Read the model definition and answer for the solid it produces. Units are mm, in the model's axes. Face numbers are marked on the shaded views. A direction names the side the tool comes from. Coordinates: 2 decimals unless noted, no trailing zeros. Write each loop counter-clockwise with the first axis right and the second up, starting at its lowest first coordinate (ties: lowest second). Pieces come first, ordered by that corner, then holes. Notation, with made-up numbers: (70.5, 21) -> (107.5, 21) arc R18 cw to (107.5, 34) -> close; hole circle Ø1 at (87, 20). An arc over 180 degrees is marked (long way). One line per item, written item: value. Start each with the question number.
1. Consider line 1 along Y through (x, z) = (-31, 1025.5); line 2 along X through (y, z) = (78.5, 673); line 3 along Y through (x, z) = (-10, 243). Determine where each line is inside the solid, lowest interval first.
2. Find section C-C, the plane y = 4. Write down the section's boundary in (x, z).
3. Given P1, Ø1.5, axis at y = 58, z = 167, coming from the -X side; P2, Ø2, axis at y = -53.5, z = 1196, coming from the +X side; P3, Ø2, axis at x = -2.5, y = 19.5, coming from the -Z side, each flat-ended and moving along its own axis, determine where each tip first touches the part or whether it passes through.
4. Find section A-A, the plane x = 38.5. Write down the section's boundary in (y, z), and give its area (3 significant figures).
5. For the marked faces 1 and 2, determine the directions among +Z, -Z, +X, -X, +Y, -Y from which every point of the face is accessible in a straight line to the end or side of a thin tool.
6. Find section B-B, the plane z = 515. Write down the section's boundary in (x, y), and give its area (3 significant figures).
Autodesk Inventor part; units mm, degrees
ref_plane "Start plane" through (0, 0, 0) normal (0, 0, 1) x (1, 0, 0)
ref_plane "End plane" through (0, 0, 1500) normal (0, 0, 1) x (1, 0, 0)
ref_plane "Work Plane4" through (-55, 0, -55) normal (0.7071, 0, -0.7071) x (-0.7071, 0, -0.7071)
ref_plane "Start plane" through (0, 0, 0) normal (0, 0, 1) x (1, 0, 0)
ref_plane "End plane" through (0, 0, 1500) normal (0, 0, 1) x (1, 0, 0)
sketch "Sketch2" plane through (0, 0, 0) normal (0, 0, 1) x (1, 0, 0)
  line L0 (-55, 100.8) -> (-14.95, 100.8)
  line L1 (-55, 110) -> (-55, 100.8)
  line L2 (55, 110) -> (-55, 110)
  line L3 (55, 100.8) -> (55, 110)
  line L4 (14.95, 100.8) -> (55, 100.8)
  line L5 (2.95, -88.8) -> (2.95, 88.8)
  line L6 (55, -100.8) -> (14.95, -100.8)
  line L7 (55, -110) -> (55, -100.8)
  line L8 (-55, -100.8) -> (-55, -110)
  line L9 (-14.95, -100.8) -> (-55, -100.8)
  line L10 (-2.95, 88.8) -> (-2.95, -88.8)
  line L11 (0, -154) -> (0, 154) construction
  line L12 (-2.95, -100.8) -> (2.95, -100.8) construction
  arc A0 (-14.95, -100.8) -> (-2.95, -88.8) centre (-14.95, -88.8) ccw
  arc A1 (-2.95, 88.8) -> (-14.95, 100.8) centre (-14.95, 88.8) ccw
  arc A2 (14.95, 100.8) -> (2.95, 88.8) centre (14.95, 88.8) ccw
  arc A3 (2.95, -88.8) -> (14.95, -100.8) centre (14.95, -88.8) ccw
  line L13 (-77, 0) -> (77, 0) construction
  line L14 (-55, -110) -> (55, -110)
  point P0 (-2.95, 100.8)
  point P1 (2.95, 100.8)
  point P2 (0, 0)
  point P3 (0, -100.8)
  point P4 (0, 0)
  dimension "d1" = 220
  dimension "d3" = 9.2
  dimension "d5" = 5.9
  dimension "d7" = 110
  dimension "d13" = 12
  dimension "d14" = 110
  dimension "d15" = 55
extrude "Body" add sketch "Sketch2" along normal up to surface (1500 mm away) from surface at 0
sketch "Sketch3" plane through (0, 0, 0) normal (0, 0, 1) x (1, 0, 0)
  line L0 (0, 0) -> (10, 0)
ref_plane "Work Plane3" through (0, 0, 0) normal (0, -1, 0) x (1, 0, 0)
ref_plane "Work Plane4" through (-55, 0, -55) normal (0.7071, 0, -0.7071) x (-0.7071, 0, -0.7071)
split "Split1" plane through (-55, 0, -55) removes the side toward (0.7071, 0, -0.7071)
ref_plane "Work Plane5" through (55, 0, -55) normal (-0.7071, 0, -0.7071) x (-0.7071, 0, 0.7071)
split "Split2" plane through (55, 0, -55) removes the side toward (-0.7071, 0, -0.7071)
ref_plane "Work Plane6" through (55, 0, 1555) normal (-0.7071, 0, 0.7071) x (0.7071, 0, 0.7071)
split "Split3" plane through (55, 0, 1555) removes the side toward (-0.7071, 0, 0.7071)
ref_plane "Work Plane7" through (-55, 0, 1555) normal (0.7071, 0, 0.7071) x (0.7071, 0, -0.7071)
split "Split4" plane through (-55, 0, 1555) removes the side toward (0.7071, 0, 0.7071)
sketch "Sketch4" plane through (0, 0, 0) normal (0, -1, 0) x (1, 0, 0)
  line L0 (-2, 0) -> (12, 0)
  line L1 (-2, 1500) -> (12, 1500)
  dimension "d19" = 1500
equation "\"d1\" = ParH"
equation "\"d3\" = t2"
equation "\"d7\" = b"
equation "\"d13\" = R1"
equation "\"d14\" = 0.5 * d1"
equation "\"d15\" = 0.5 * d7"
equation "\"d8\" = G_L"
equation "\"b\" = 110"
equation "\"ParH\" = 220"
equation "\"R1\" = 12"
equation "\"G_L\" = d19"
equation "\"t1\" = 5.9"
equation "\"t2\" = 9.2"
equation "\"G_OFFSET_START\" = 0"
equation "\"G_OFFSET_END\" = 0"
properties part number "DIN 1025 - IPE 220-1500" material "Steel, Mild"
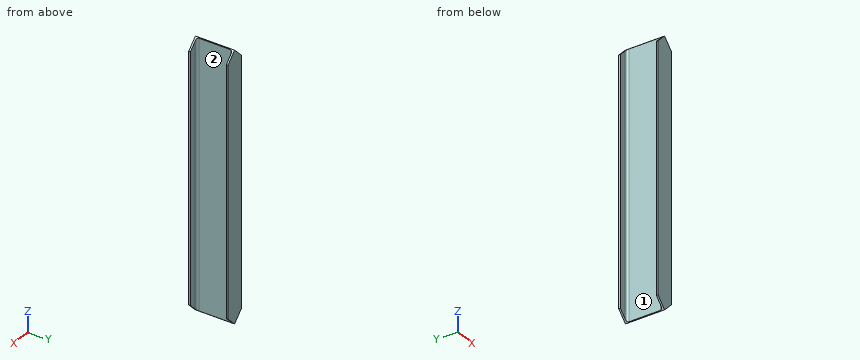
Answer block:
1. line 1: y = -110 to -100.8, 100.8 to 110
1. line 2: x = -2.95 to 2.95
1. line 3: y = -110 to -99.73, 99.73 to 110
2. outline: (-2.95, 2.95) -> (0, 0) -> (2.95, 2.95) -> (2.95, 1497.05) -> (0, 1500) -> (-2.95, 1497.05) -> close
3. P1: stops at x = -2.95
3. P2: stops at x = 2.95
3. P3: stops at z = 1.5
4. outline: (-110, 38.5) -> (-100.8, 38.5) -> (-100.8, 1461.5) -> (-110, 1461.5) -> close; (100.8, 38.5) -> (110, 38.5) -> (110, 1461.5) -> (100.8, 1461.5) -> close
4. area: 26,200 mm2
5. face 1: +Z, -Z, -X
5. face 2: +Z, -Z, +X
6. outline: (-55, -110) -> (55, -110) -> (55, -100.8) -> (14.95, -100.8) arc R12 cw to (2.95, -88.8) -> (2.95, 88.8) arc R12 cw to (14.95, 100.8) -> (55, 100.8) -> (55, 110) -> (-55, 110) -> (-55, 100.8) -> (-14.95, 100.8) arc R12 cw to (-2.95, 88.8) -> (-2.95, -88.8) arc R12 cw to (-14.95, -100.8) -> (-55, -100.8) -> close
6. area: 3,340 mm2
